from build123d import *
from build123d.topology import SkipClean

# Parameters (mm, degrees)
SKETCH_1_R               = 36
SKETCH_1_R_2             = 4.15
EXTRUDE_1_DEPTH          = 2
SKETCH_2_W               = 45
SKETCH_2_H               = 45
EXTRUDE_2_DEPTH          = 25
SKETCH_3_R               = 36
SKETCH_3_R_2             = 4.15
EXTRUDE_3_DEPTH          = 2
EXTRUDE_4_DEPTH          = 25
CUT_EXTRUDE_1_DEPTH      = 50
EXTRUDE_6_DEPTH          = 25
CUT_EXTRUDE_3_DEPTH      = 38.25
CUT_EXTRUDE_3_DEPTH_BACK = 0.25
CUT_EXTRUDE_4_DEPTH      = 50
CUT_EXTRUDE_4_DEPTH_BACK = 4
SKETCH_20_W              = 45
SKETCH_20_H              = 45
EXTRUDE_7_DEPTH          = 13
FILLET_1_R               = 3
FILLET_2_R               = 1
SKETCH_22_R              = 36
CUT_EXTRUDE_6_DEPTH      = 40
SKETCH_24_R              = 5
CUT_EXTRUDE_7_DEPTH      = 2
FILLET_3_R               = 4


with BuildPart() as part:
    # Sketch 1 → Extrude 1 (new body)
    with BuildSketch(Plane.XY):
        Circle(SKETCH_1_R)
        with Locations((0, 30.5)):
            Circle(SKETCH_1_R_2, mode=Mode.SUBTRACT)
        with Locations((-30.5, 0)):
            Circle(SKETCH_1_R_2, mode=Mode.SUBTRACT)
        with Locations((0, -30.5)):
            Circle(SKETCH_1_R_2, mode=Mode.SUBTRACT)
        with Locations((30.5, 0)):
            Circle(SKETCH_1_R_2, mode=Mode.SUBTRACT)
    extrude(amount=EXTRUDE_1_DEPTH)

    # Sketch 2 → Extrude 2 (add)
    with BuildSketch(Plane.XY.offset(2)):
        Rectangle(SKETCH_2_W, SKETCH_2_H)
    extrude(amount=EXTRUDE_2_DEPTH)

    # Sketch 3 → Extrude 3 (add)
    with BuildSketch(Plane.XY.offset(27)):
        Circle(SKETCH_3_R)
        with Locations((0, 30.5)):
            Circle(SKETCH_3_R_2, mode=Mode.SUBTRACT)
        with Locations((0, -30.5)):
            Circle(SKETCH_3_R_2, mode=Mode.SUBTRACT)
        with Locations((-30.5, 0)):
            Circle(SKETCH_3_R_2, mode=Mode.SUBTRACT)
        with Locations((30.5, 0)):
            Circle(SKETCH_3_R_2, mode=Mode.SUBTRACT)
    extrude(amount=EXTRUDE_3_DEPTH)

    # Sketch 8 → Extrude 4 (add)
    with SkipClean():  # the faces are left unmerged after this step: merging them gives an invalid solid
        with BuildSketch(Plane.XY.offset(29)):
            with BuildLine():
                Line((-13.435028843, 13.435028843), (0, 0))
                Line((0, 0), (17.67766953, 17.67766953))
                Line((17.67766953, 17.67766953), (4.242640687, 31.112698372))
                Line((4.242640687, 31.112698372), (4.120861375, 30.990919061))
                ThreePointArc((4.120861375, 30.990919061), (4.142708939, 30.745891533), (4.15, 30.5))
                ThreePointArc((4.15, 30.5), (2.755466013, 27.396790846), (-0.490919061, 26.379138625))
                Line((-0.490919061, 26.379138625), (-13.435028843, 13.435028843))
            make_face()
            with BuildLine():
                Line((17.67766953, 17.67766953), (0, 0))
                Line((0, 0), (13.435028843, -13.435028843))
                Line((13.435028843, -13.435028843), (26.379138625, -0.490919061))
                ThreePointArc((26.379138625, -0.490919061), (27.565506858, 2.934493142), (30.990919061, 4.120861375))
                Line((30.990919061, 4.120861375), (31.112698372, 4.242640687))
                Line((31.112698372, 4.242640687), (17.67766953, 17.67766953))
            make_face()
            with BuildLine():
                Line((-17.67766953, -17.67766953), (0, 0))
                Line((0, 0), (-13.435028843, 13.435028843))
                Line((-13.435028843, 13.435028843), (-26.379138625, 0.490919061))
                ThreePointArc((-26.379138625, 0.490919061), (-26.357291061, 0.245891533), (-26.35, 0))
                ThreePointArc((-26.35, 0), (-27.744533987, -3.103209154), (-30.990919061, -4.120861375))
                Line((-30.990919061, -4.120861375), (-31.112698372, -4.242640687))
                Line((-31.112698372, -4.242640687), (-17.67766953, -17.67766953))
            make_face()
            with BuildLine():
                Line((13.435028843, -13.435028843), (0, 0))
                Line((0, 0), (-17.67766953, -17.67766953))
                Line((-17.67766953, -17.67766953), (-4.242640687, -31.112698372))
                Line((-4.242640687, -31.112698372), (-4.120861375, -30.990919061))
                ThreePointArc((-4.120861375, -30.990919061), (-2.934493142, -27.565506858), (0.490919061, -26.379138625))
                Line((0.490919061, -26.379138625), (13.435028843, -13.435028843))
            make_face()
        extrude(amount=EXTRUDE_4_DEPTH)

    # Sketch 12 → Cut-Extrude 1 (cut)
    with BuildSketch(Plane(origin=(13.435028843, -13.435028843, 0), x_dir=(0, 0, -1), z_dir=(0.7071067811865477, -0.7071067811865474, 0))):
        Polygon((-32.347132197, -18.305735607), (-50.652867803, 18.305735607), (-54, 18.305735607), (-54, -18.305735607), align=None)
        Polygon((-50.652867803, 18.305735607), (-54, 25), (-54, 18.305735607), align=None)
        Polygon((-29, -25), (-32.347132197, -18.305735607), (-54, -18.305735607), (-54, -25), align=None)
    extrude(amount=-CUT_EXTRUDE_1_DEPTH, mode=Mode.SUBTRACT)

    # Sketch 16 → Extrude 6 (add)
    with SkipClean():  # the faces are left unmerged after this step: merging them gives an invalid solid
        with BuildSketch(Plane.XY.offset(29)):
            Polygon((-24.04163056, 2.828427125), (-13.435028843, 13.435028843), (-2.828427125, 24.04163056), (-4.949747468, 26.162950904), (-26.162950904, 4.949747468), align=None)
            Polygon((24.04163056, -2.828427125), (13.435028843, -13.435028843), (2.828427125, -24.04163056), (4.949747468, -26.162950904), (26.162950904, -4.949747468), align=None)
        extrude(amount=EXTRUDE_6_DEPTH)

    # Sketch 17 → Cut-Extrude 3 (cut, two sides: drawn at the far end of the back side and taken through both)
    with SkipClean():  # the faces are left unmerged after this step: merging them gives an invalid solid
        with BuildSketch(Plane(origin=(-13.435028843, 13.435028843, 0), x_dir=(0, 0, -1), z_dir=(0.7071067811865477, -0.7071067811865474, 0)).offset(-CUT_EXTRUDE_3_DEPTH_BACK)):
            Polygon((-49, 15), (-34, -15), (-54, -15), (-54, 15), align=None)
        extrude(amount=CUT_EXTRUDE_3_DEPTH + CUT_EXTRUDE_3_DEPTH_BACK, mode=Mode.SUBTRACT)

    # Sketch 18 → Cut-Extrude 4 (cut, two sides: drawn at the far end of the back side and taken through both)
    with SkipClean():  # the faces are left unmerged after this step: merging them gives an invalid solid
        with BuildSketch(Plane(origin=(-13.611805538, 13.611805538, 0), x_dir=(0, 0, -1), z_dir=(0.7071067811865477, -0.7071067811865474, 0)).offset(-CUT_EXTRUDE_4_DEPTH_BACK)):
            Polygon((-44.201018115, 13.183932796), (-38.387241373, 1.556379313), (-36.5, 2.5), (-42.313776741, 14.127553483), align=None)
            Polygon((-36.5, 2.5), (-38.387241373, 1.556379313), (-32.573464632, -10.07117417), (-30.686223259, -9.127553483), align=None)
            Polygon((-29, -8.284441854), (-40.83096799, 14.868957859), (-42.313776741, 14.127553483), (-36.5, 2.5), (-30.686223259, -9.127553483), align=None)
        extrude(amount=CUT_EXTRUDE_4_DEPTH + CUT_EXTRUDE_4_DEPTH_BACK, mode=Mode.SUBTRACT)

    # Sketch 20 → Extrude 7 (add)
    with SkipClean():  # the faces are left unmerged after this step: merging them gives an invalid solid
        with BuildSketch(Plane(origin=(0, 0, 0), x_dir=(-1, 0, 0), z_dir=(0, 0, -1))):
            Rectangle(SKETCH_20_W, SKETCH_20_H)
        extrude(amount=EXTRUDE_7_DEPTH)

    # Fillet 1
    fillet_1_edges = [part.edges().sort_by_distance(p)[0] for p in [
        (17.67766953, 17.67766953, 54),
    ]]
    fillet(fillet_1_edges, radius=FILLET_1_R)

    # Fillet 2
    fillet_2_edges = [part.edges().sort_by_distance(p)[0] for p in [
        (-13.611805538, 13.611805538, 54),
        (13.611805538, -13.611805538, 54),
    ]]
    fillet(fillet_2_edges, radius=FILLET_2_R)

    # Sketch 22 → Cut-Extrude 6 (cut)
    with SkipClean():  # the faces are left unmerged after this step: merging them gives an invalid solid
        with BuildSketch(Plane(origin=(0, 0, -13), x_dir=(-1, 0, 0), z_dir=(0, 0, -1))):
            with Locations(Location((0, 0, 0), (0, 0, 180))):
                Circle(SKETCH_22_R)
        extrude(amount=-CUT_EXTRUDE_6_DEPTH, mode=Mode.SUBTRACT)

    # Sketch 24 → Cut-Extrude 7 (cut)
    with SkipClean():  # the faces are left unmerged after this step: merging them gives an invalid solid
        with BuildSketch(Plane(origin=(0, 0, 27), x_dir=(-1, 0, 0), z_dir=(0, 0, -1))):
            with Locations((30.5, 11.72)):
                Circle(SKETCH_24_R)
        extrude(amount=-CUT_EXTRUDE_7_DEPTH, mode=Mode.SUBTRACT)

    # Fillet 3
    fillet_3_edges = [part.edges().sort_by_distance(p)[0] for p in [
        (-34.808921563, 9.183625626, 28),
        (-32.001676968, 16.489168301, 28),
    ]]
    fillet(fillet_3_edges, radius=FILLET_3_R)


solid = part.part
CAD build for the part. Positions are in the model's coordinates, mm. A direction names the side the tool comes from. Round coordinates to 2 decimals unless told otherwise and drop trailing zeros. Use a Markdown table: item, result. Add a question column.
1. Drill centre lines: probe 1 along X at (y, z) = (0, 28.45); probe 2 along Z at (x, y) = (5, -30.5). Where is each one in solid material? Low to high.
2. Pull direction Y, two halves, no side cores. Call faces 6 (the face through (-25.19, 1.68, 30.91)), 7 (the face through (-1, 1, 27)), 8 (the face through (-3.874, 25.087, 41.325)): released by +Y, released by -Y, zero draft, split by the parting line, or undercut.
3. 3-axis set-ups, long thin cutter, end or side, ignore diameter. For faces 1 (the face through (-15.41, 15.7, 41.32)), 2 (the face through (-25.117, 3.904, 41.325)), 3 (the face through (1.64, -25.23, 30.91)), 4 (the face through (25.117, -3.904, 41.325)), 5 (the face through (1.996, 2.431, 34.833)): which of +Z, -Z, +X, -X, +Y, -Y reach the whole face in a straight line?
4. Flat gauge pins, fed straight in: P1, Ø1, axis at x = -15, z = 46, coming from the +Y side; P2, Ø3, axis at y = 27, z = 47, coming from the -X side; P3, Ø6, axis at y = -13, z = 45.5, coming from the -X side. Where does each tip first touch, or does it go through?
Reply:
| question | item | result |
|---|---|---|
| 1 | probe 1 | x = -36 to -34.65, -26.35 to 26.35, 34.65 to 36 |
| 1 | probe 2 | z = 27 to 29 |
| 2 | face 6 | undercut |
| 2 | face 7 | zero draft |
| 2 | face 8 | released by +Y |
| 3 | face 1 | +Z, -X, +Y |
| 3 | face 2 | +Z, -X |
| 3 | face 3 | +Z, -Y |
| 3 | face 4 | +Z, +X |
| 3 | face 5 | none |
| 4 | P1 | stops at y = 16.61 |
| 4 | P2 | stops at x = -5.61 |
| 4 | P3 | stops at x = 11.22 |
